Part model, mm, in its own coordinate system. A direction names the side the tool comes from. Coordinates: 2 decimals unless noted, no trailing zeros. Loops run counter-clockwise (first coordinate to the right, second up) from the corner with the lowest first, then second, coordinate; pieces in that order, holes last. Notation, with made-up numbers: M 39.5,-10 L 95.5,-10 A16 ccw 95.5,0 Z; hole C -39,10 d7. An arc over 180 degrees is marked long. Use a Markdown table: item, result. Add a question column.
1) Band-saw the part on C-C (z = -3.25). List the corners of the cut face in (x, y).
2) Band-saw the part on B-B (y = 21.5). List the corners of the cut face in (x, z), plus the area to 3 significant figures.
3) Band-saw the part on A-A (x = 3). List the corners of the cut face in (y, z).
4) Wall check: probe 1 along Z at (x, y) = (-10, 15); probe 2 along Y at (x, z) = (8.5, -9.25). Give the ranges that are in metal, low to high. Write a range as from..to.
5) Band-saw the part on D-D (x = -12.5). List the corners of the cut face in (y, z).
6) Pin check, flat tips, straight feed: pin 1 Ø1 at (x, z) = (-8, -6) entering from +Y; pin 2 Ø3 at (x, y) = (-9, -16) entering from -Z. Stop position of each tip, or through.
7) Pull direction Y, two halves, no side cores. Call faces 4 (the flat face through (-8.56, 22, -7)), 5 (the cylindrical face through (29.63, 26.28, 0.01)), 6 (the flat face through (2, 18.034, -7)): released by +Y, released by -Y, zero draft, split by the parting line, or undercut.
8) Tool access for faces 1 (the flat face through (12.319, 22, -7)), 2 (the flat face through (2, 27.051, -7)), 3 (the cylindrical face through (-29.32, -24.9, 0.01)): list every direction of +Z, -Z, +X, -X, +Y, -Y with a clear straight run to the whole face (end or side of a thin tool).
from build123d import *

# Parameters (mm, degrees)
SKETCH1_W           = 61.468
SKETCH1_H           = 56.642
BOSS_EXTRUDE1_DEPTH = 0.8255
SKETCH6_W           = 20.8788
SKETCH6_H           = 9.017
BOSS_EXTRUDE3_DEPTH = 13.081
SKETCH3_R           = 1.4224
CUT_EXTRUDE1_DEPTH  = 45.313537672


with BuildPart() as part:
    # Sketch1 → Boss-Extrude1 (new, symmetric)
    with BuildSketch(Plane.XY):
        Rectangle(SKETCH1_W, SKETCH1_H)
    extrude(amount=BOSS_EXTRUDE1_DEPTH, both=True)

    # Sketch6 → Boss-Extrude3 (add)
    with BuildSketch(Plane(origin=(0, 0, -0.8255), x_dir=(-1, 0, 0), z_dir=(0, 0, -1))):
        with Locations((-1.8796, 22.5425)):
            Rectangle(SKETCH6_W, SKETCH6_H)
    extrude(amount=BOSS_EXTRUDE3_DEPTH)

    # Sketch3 → Cut-Extrude1 (cut, through all)
    with BuildSketch(Plane.XY.offset(0.8255)):
        with Locations((-28.2702, 25.8572)):
            Circle(SKETCH3_R)
        with Locations((28.2702, 25.8572)):
            Circle(SKETCH3_R)
        with Locations((28.2702, -25.8572)):
            Circle(SKETCH3_R)
        with Locations((-28.2702, -25.8572)):
            Circle(SKETCH3_R)
    extrude(amount=-CUT_EXTRUDE1_DEPTH, mode=Mode.SUBTRACT)


solid = part.part
Entries:
| question | item | result |
|---|---|---|
| 1 | outline | M -8.56,18.03 L 12.32,18.03 L 12.32,27.05 L -8.56,27.05 Z |
| 2 | outline | M -30.73,-0.83 L -8.56,-0.83 L -8.56,-13.91 L 12.32,-13.91 L 12.32,-0.83 L 30.73,-0.83 L 30.73,0.83 L -30.73,0.83 Z |
| 2 | area | 375 mm2 |
| 3 | outline | M -28.32,-0.83 L 18.03,-0.83 L 18.03,-13.91 L 27.05,-13.91 L 27.05,-0.83 L 28.32,-0.83 L 28.32,0.83 L -28.32,0.83 Z |
| 4 | probe 1 | -0.83..0.83 |
| 4 | probe 2 | 18.03..27.05 |
| 5 | outline | M -28.32,-0.83 L 28.32,-0.83 L 28.32,0.83 L -28.32,0.83 Z |
| 6 | pin 1 | y = 27.05 |
| 6 | pin 2 | z = -0.83 |
| 7 | face 4 | zero draft |
| 7 | face 5 | undercut |
| 7 | face 6 | released by -Y |
| 8 | face 1 | -Z, +X, +Y, -Y |
| 8 | face 2 | -Z, +X, -X, +Y |
| 8 | face 3 | +Z, -Z |
